Autodesk Inventor part; units mm, degrees
ref_plane "Work Plane1" through (10.95, 0, 0) normal (0, 0, -1) x (1, 0, 0)
ref_plane "YZ Plane" through (0, 0, 0) normal (1, 0, 0) x (0, 1, 0)
ref_plane "XZ Plane" through (0, 0, 0) normal (0, 1, 0) x (-1, 0, 0)
sketch "Sketch1" plane through (0, 0, 0) normal (0, 0, 1) x (1, 0, 0)
  line L0 (-3.825, 0) -> (-3.825, 4.5101)
  line L1 (0, 7.3) -> (0, 4)
  line L2 (13, 4) -> (35, 4)
  line L3 (35, 4) -> (35, 0)
  line L4 (35, 0) -> (-3.825, 0)
  arc A0 (0, 7.3) -> (-2.2876, 7.8071) centre (-1.2, 7.3) ccw
  line L5 (0, -1.745) -> (0, 10.4702)
  line L6 (-11.59, 0) -> (42.765, 0)
  line L7 (0, 4) -> (0.0001, 4)
  line L8 (0.0001, 4) -> (0.0001, 4)
  line L9 (0.0001, 4) -> (12.2332, 4)
  line L10 (12.2332, 4) -> (13, 4)
  line L11 (-3.825, 4.5101) -> (-2.2876, 7.8071)
  line L12 (0.0001, 4) -> (13, 4) construction
  line L13 (13, 4) -> (13, 0) construction
  dimension "d0" = 1.2
  dimension "d1" = 35
  dimension "d2" = 22
  dimension "d3" = 17
  dimension "d4" = 8
  dimension "d5" = 3.825
  dimension "d15" = 8
  dimension "d16" = 8
  dimension "d17" = 0.0001
  dimension "d18" = 0.7668
  dimension "d19" = 25
revolve "Body" add sketch "Sketch1" angle 360 about axis through (35, 0, 0) along (-1, 0, 0)
sketch "Sketch2" plane through (0, 0, 0) normal (1, 0, 0) x (0, 0, -1)
  line L0 (5, 2.8868) -> (5, -2.8868)
  line L1 (5, -2.8868) -> (0, -5.7735)
  line L2 (0, -5.7735) -> (-5, -2.8868)
  line L3 (-5, -2.8868) -> (-5, 2.8868)
  line L4 (-5, 2.8868) -> (0, 5.7735)
  line L5 (0, 5.7735) -> (5, 2.8868)
  point P0 (0, 0)
  point P1 (0, 0)
  dimension "d23" = 10
extrude "Head" add sketch "Sketch2" against normal blind 8.5
sketch "Sketch3" plane through (0, 0, 0) normal (0, 0, 1) x (1, 0, 0)
  line L0 (-8.5, 4.75) -> (-8.5, 5.7735)
  line L1 (-8.5, 5.7735) -> (-7.9091, 5.7735)
  line L2 (-7.9091, 5.7735) -> (-8.5, 4.75)
  line L3 (-9.5528, 0) -> (-2.183, 0)
  line L4 (-8.5, 5.7735) -> (-8.5, 2.8868)
  line L5 (-3.2359, 5.7735) -> (-8.5, 5.7735)
  point P0 (-8.5, 2.8868)
  dimension "d8" = 30
  dimension "d22" = 9.5
revolve "Chamfer1" cut sketch "Sketch3" angle 360 about axis through (-10, 0, 0) along (1, 0, 0)
thread "Thread"
chamfer "Chamfer2" distance 0.7668 distance2 0.7668 1 edges at (35, -4, 0) measured on face at (35, 1.5232, 1.2467)
ref_plane "Work Plane1" through (10.95, 0, 0) normal (0, 0, -1) x (1, 0, 0)
equation "\"d0\" = PHH"
equation "\"d1\" = NLG"
equation "\"d2\" = GEL"
equation "\"d3\" = LADI"
equation "\"d4\" = GD"
equation "\"d5\" = 0.45 * KOH"
equation "\"d15\" = SD2"
equation "\"d16\" = BDM"
equation "\"d18\" = GAL"
equation "\"d19\" = KEWI"
equation "\"d23\" = SW"
equation "\"d6\" = KOH"
equation "\"d8\" = ANG1"
equation "\"d22\" = SW0"
equation "\"d10\" = GEL"
equation "\"d13\" = -0.5 * SPD + 0.5 * GD"
equation "\"d14\" = GUL"
equation "\"NLG\" = 35"
equation "\"GD\" = NND"
equation "\"BDM\" = NND"
equation "\"KOH\" = 8.5"
equation "\"GEL\" = 22"
equation "\"LADI\" = 17"
equation "\"SW\" = 10"
equation "\"PHH\" = RR"
equation "\"SW0\" = 9.5"
equation "\"SPD\" = NND - 1.2269 * PTC"
equation "\"SD2\" = NND"
equation "\"SD\" = 0"
equation "\"ANG1\" = 30deg"
equation "\"KEWI\" = 25deg"
equation "\"GAL\" = 0.61345 * PTC"
equation "\"GUL\" = 0.61345 * PTC"
equation "\"PTC\" = 1.25"
equation "\"THREADDIA\" = 8"
equation "\"E0\" = 1.155 * SW"
equation "\"TOA\" = 30deg"
equation "\"NND\" = 8"
equation "\"GD1\" = THREADDIA - 1.2269 * PTC"
equation "\"KOH1\" = 3.8"
equation "\"RR\" = 1.2"
properties part number "ISO 4162 - M8 x 35" material "Stainless Steel"
Design review of the part built by this model. Coordinates are the model's own, in mm. A direction names the side the tool comes from. Round coordinates to 2 decimals unless told otherwise and drop trailing zeros. Write each loop counter-clockwise with the first axis right and the second up, starting at its lowest first coordinate (ties: lowest second). Pieces come first, ordered by that corner, then holes. Notation, with made-up numbers: M 23.25,74.5 L 45.25,74.5 A16 ccw 45.25,103.5 Z; hole C 11,83 d6. An arc over 180 degrees is marked long. One line per item, written item: value. Start each with the question number.
1. For faces 1 (the face through (-5.76, 4.31, 2.535)), 2 (the face through (0, 3, 3)), 3 (the face through (-5.76, -4.31, -2.535)), 4 (the face through (-5.76, -4.35, 2.465)), 5 (the face through (-5.76, 4.35, -2.465)), list the 3-axis set-ups (+Z, -Z, +X, -X, +Y, -Y) from which the entire face can be reached by the end or side of a thin tool; tool diameter is ignored.
2. Take a section at A-A on y = 0. State the section outline as (x, z) points, then the cut area to 3 significant figures.
3. Clearance check with flat-ended pins moving along their axes: P1, Ø8, axis at x = 9.5, z = -1.5, coming from the +Y side; P2, Ø2, axis at x = 17.5, y = -4.5, coming from the +Z side; P3, Ø6, axis at y = -3, z = 5.5, coming from the +X side; P4, Ø1.5, axis at x = 19.5, z = 6.5, coming from the +Y side. State where each tip first meets the part, or that it passes through.
4. Take a section at B-B on x = 26.5. State the section outline as (y, z) points, then the cut area to 3 significant figures.
5. To check wall thickness, follow probe 1 along Z at (x, y) = (33, -0.25); probe 2 along X at (y, z) = (-4.25, 2); probe 3 along Z at (x, y) = (-4, -1.75). State the ranges of each line that lie inside material, in increasing order. Write a range as from..to.
Computed:
1. face 1: +Z, -X, +Y
1. face 2: +X
1. face 3: -Z, -X, -Y
1. face 4: +Z, -X, -Y
1. face 5: -Z, -X, +Y
2. outline: M -8.5,-4.75 L -8.36,-5 L -3.6,-5 L -2.29,-7.81 A1.2 ccw 0,-7.3 L 0,-4 L 34.23,-4 L 35,-3.23 L 35,3.23 L 34.23,4 L 0,4 L 0,7.3 A1.2 ccw -2.29,7.81 L -3.6,5 L -8.36,5 L -8.5,4.75 Z
2. area: 383 mm²
3. P1: stops at y = 4
3. P2: stops at z = 1.94
3. P3: stops at x = 34.97
3. P4: passes through
4. outline: C 0,0 d8
4. area: 50.3 mm²
5. probe 1: z = -3.99..3.99
5. probe 2: x = -8.5..0
5. probe 3: z = -5..5
